Study the drawing (mm; zero at the part's minimum x, y, z) and answer. Coordinates: 2 decimals unless noted, no trailing zeros. Loops run counter-clockwise (first coordinate to the right, second up) from the corner with the lowest first, then second, coordinate; pieces in that order, holes last. Notation, with made-up numbers: (59.25, -21) - (105.25, -21) arc R13 ccw to (105.25, 0) - close; hole circle Ø9 at (-8.5, 70). An arc over 180 degrees is marked (long way). Put each result on its own line as item: value.
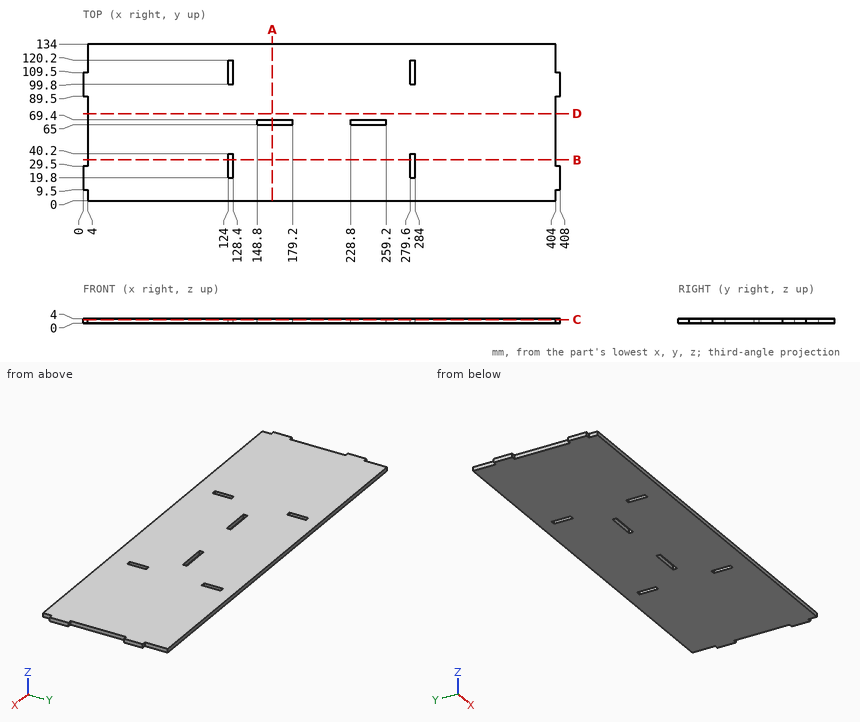
1) The part is cut by section C-C (z = 3.15). State how many separate pieces and enclosed holes the cut face has, and give its area (3 significant figures).
Found:
separate pieces: 1
enclosed holes: 6
area: 53,300 mm^2
2) The part is cut by section B-B (y = 35). Give the vertices of the cut face in (x, z), and give its area (3 significant figures).
Found:
outline: (4, 0) - (124, 0) - (124, 4) - (4, 4) - close; (128.4, 0) - (279.6, 0) - (279.6, 4) - (128.4, 4) - close; (284, 0) - (404, 0) - (404, 4) - (284, 4) - close
area: 1,560 mm^2
3) This flat-tipped pin is pushed along its axis until it touches: pin 1 (2 mm diameter, centred on y = 67.5, z = 1.5, fed in from +X). Where does it stop, or does it pass through?
Found:
pin 1: stops at x = 404
4) The part is cut by section A-A (x = 162). Give the vertices of the cut face in (y, z).
Found:
outline: (0, 0) - (65, 0) - (65, 4) - (0, 4) - close; (69.4, 0) - (134, 0) - (134, 4) - (69.4, 4) - close
5) Straight lines are drawn through the part: L1, parallel to X at y = 26.5, z = 0.4; L2, parallel to X at y = 120, z = 1.6; L3, parallel to Y at x = 238, z = 3. For each, find the intervals that lie inside material, in ascending order. Write a range as [from, to].
Found:
L1: x = [0, 124], [128.4, 279.6], [284, 408]
L2: x = [4, 124], [128.4, 279.6], [284, 404]
L3: y = [0, 65], [69.4, 134]
6) The part is cut by section D-D (y = 74.5). Give the vertices of the cut face in (x, z), and give its area (3 significant figures).
Found:
outline: (4, 0) - (404, 0) - (404, 4) - (4, 4) - close
area: 1,600 mm^2
